```python
from build123d import *

# Parameters (mm, degrees)
SKETCH1_W           = 152.4
SKETCH1_H           = 152.4
SKETCH1_R           = 63.5
BOSS_EXTRUDE1_DEPTH = 1.5875
SKETCH2_R           = 66.04
SKETCH2_R_2         = 63.5
BOSS_EXTRUDE2_DEPTH = 4.445
SKETCH3_R           = 3.175
CUT_EXTRUDE1_DEPTH  = 1.5875


with BuildPart() as part:
    # Sketch1 → Boss-Extrude1 (new body)
    with BuildSketch(Plane.XY):
        Rectangle(SKETCH1_W, SKETCH1_H)
        Circle(SKETCH1_R, mode=Mode.SUBTRACT)
    extrude(amount=BOSS_EXTRUDE1_DEPTH)

    # Sketch2 → Boss-Extrude2 (add)
    with BuildSketch(Plane.XY.offset(1.5875)):
        Circle(SKETCH2_R)
        Circle(SKETCH2_R_2, mode=Mode.SUBTRACT)
    extrude(amount=BOSS_EXTRUDE2_DEPTH)

    # Sketch3 → Cut-Extrude1 (cut)
    with BuildSketch(Plane.XY.offset(1.5875)):
        with Locations((66.8782, -66.8782)):
            Circle(SKETCH3_R)
        with Locations((-66.8782, -66.8782)):
            Circle(SKETCH3_R)
        with Locations((-66.8782, 66.8782)):
            Circle(SKETCH3_R)
        with Locations((66.8782, 66.8782)):
            Circle(SKETCH3_R)
    extrude(amount=-CUT_EXTRUDE1_DEPTH, mode=Mode.SUBTRACT)


solid = part.part
```
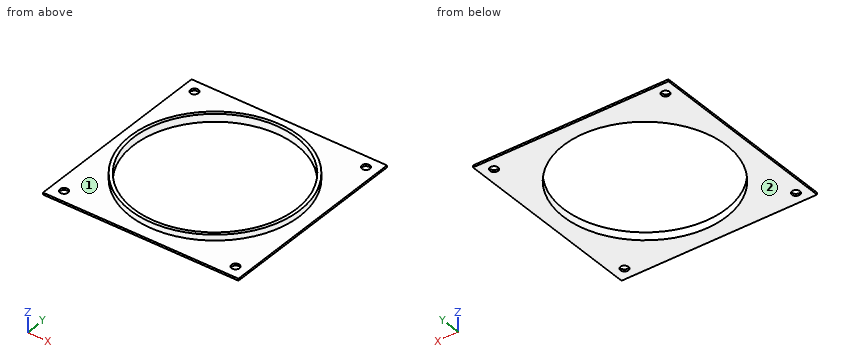
The model under review builds one solid part; all positions refer to its coordinate system, in mm. Face numbers are marked on the shaded views. A direction names the side the tool comes from. Give positions to 0.01 mm unless a question says otherwise; leave off trailing zeros. Write each loop counter-clockwise with the first axis right and the second up, starting at its lowest first coordinate (ties: lowest second). Pieces come first, ordered by that corner, then holes. Notation, with made-up numbers: (66.5, 86) - (92.5, 86) arc R19 cw to (92.5, 103) - close; hole circle Ø7 at (-16, -21). An arc over 180 degrees is marked (long way). Answer in a Markdown table with one row per item. Add a question column.
1. Wall thickness on line 1 along Y through (x, z) = (0, 1.5); line 2 along X through (y, z) = (34, 5.5); line 3 along Y through (x, z) = (37, 0.5): over which ranges is each line inside the solid? List them lowest first. Write a range as [from, to].
2. Insertion check: P1, Ø1.5, axis at x = 41, z = 4.5, coming from the +Y side; P2, Ø1.5, axis at y = 55, z = 4.5, coming from the +X side; P3, Ø3, axis at x = -24, z = 3.5, coming from the -Y side; P4, Ø4, axis at x = 66.88, y = -66.88, coming from the -Z side. Each pin has a flat end and moves straight along its axis. Give the tip position at first contact, or say it passes through.
3. We need section C-C on z = 5. Write out the cut boundary in (x, y), then the cut area to 3 significant figures.
4. Tool access review of the marked faces 1 and 2: name each direction out of +Z, -Z, +X, -X, +Y, -Y from which nothing blocks a thin tool from reaching the whole face with its end or side.
5. We need section A-A on y = 0. Write out the cut boundary in (x, z).
Ans:
| question | item | result |
|---|---|---|
| 1 | line 1 | y = [-76.2, -63.5], [63.5, 76.2] |
| 1 | line 2 | x = [-56.62, -53.63], [53.63, 56.62] |
| 1 | line 3 | y = [-76.2, -51.61], [51.61, 76.2] |
| 2 | P1 | stops at y = 52.36 |
| 2 | P2 | stops at x = 37.66 |
| 2 | P3 | stops at y = -62.09 |
| 2 | P4 | passes through |
| 3 | outline | circle Ø132.08 at (0, 0); hole circle Ø127 at (0, 0) |
| 3 | area | 1,030 mm^2 |
| 4 | face 1 | +Z |
| 4 | face 2 | -Z, +X, -X, +Y, -Y |
| 5 | outline | (-76.2, 0) - (-63.5, 0) - (-63.5, 6.03) - (-66.04, 6.03) - (-66.04, 1.59) - (-76.2, 1.59) - close; (63.5, 0) - (76.2, 0) - (76.2, 1.59) - (66.04, 1.59) - (66.04, 6.03) - (63.5, 6.03) - close |
